from build123d import *

# Parameters (mm, degrees)
F0_W     = 56
F0_H     = 30
F0_R     = 5
F1_DEPTH = 15
F2_W     = 56
F2_H     = 15
F3_DEPTH = 18
F4_W     = 15
F4_H     = 5
F5_DEPTH = 25
F6_W     = 2
F6_H     = 15
F7_DEPTH = 20
F8_W     = 12
F8_H     = 15
F9_DEPTH = 20


with BuildPart() as f1:
    # F0 (on Top) → F1 (new body)
    with BuildSketch(Plane.XY):
        Rectangle(F0_W, F0_H)
        Circle(F0_R, mode=Mode.SUBTRACT)
    extrude(amount=F1_DEPTH)

    # F2 (on face) → F3 (cut)
    with BuildSketch(Plane.XZ.offset(15)):
        with Locations((0, 7.5)):
            Rectangle(F2_W, F2_H)
    extrude(amount=-F3_DEPTH, mode=Mode.SUBTRACT)

    # F4 (on face) → F5 (cut)
    with BuildSketch(Plane(origin=(0, 15, 0), x_dir=(-1, 0, 0), z_dir=(0, 1, 0))):
        with Locations((17.5, 7.5)):
            Rectangle(F4_W, F4_H)
    extrude(amount=-F5_DEPTH, mode=Mode.SUBTRACT)

    # F6 (on face) → F7 (cut)
    with BuildSketch(Plane(origin=(-28, 0, 0), x_dir=(0, -1, 0), z_dir=(-1, 0, 0))):
        with Locations((-4, 7.5)):
            Rectangle(F6_W, F6_H)
    extrude(amount=-F7_DEPTH, mode=Mode.SUBTRACT)

    # F8 (on face) → F9 (cut)
    with BuildSketch(Plane.YZ.offset(28)):
        with Locations((9, 7.5)):
            Rectangle(F8_W, F8_H)
    extrude(amount=-F9_DEPTH, mode=Mode.SUBTRACT)


solid = f1.part
Can you work these out from the model? Positions are in its coordinate system, mm. A direction names the side the tool comes from. Round coordinates to 2 decimals unless told otherwise and drop trailing zeros. Order: outer loops, then holes, each group sorted by start corner. A loop starts at its lowest first (then second) coordinate and runs counter-clockwise, first axis right, second up. Notation, with made-up numbers: M 35.25,7.25 L 40.25,7.25 A8 cw 40.25,14.25 Z; hole C 85.25,45.25 d5. An arc over 180 degrees is marked long. Use a Markdown table: item, result.
1) I'm going to push flat-ended pins straight in: P1, Ø2, axis at x = -22.5, z = 12.5, coming from the -Y side; P2, Ø1.6, axis at y = 4, z = 5, coming from the -X side; P3, Ø1, axis at x = -1.5, z = 8.5, coming from the -Y side. Where does each tip first touch, or does it pass through?
Geometry says:
| item | result |
|---|---|
| P1 | stops at y = 5 |
| P2 | stops at x = -8 |
| P3 | stops at y = 4.58 |
2) Imagine slicing it at A-A (x = -18). List the corners of the cut face in (y, z) for me.
Geometry says:
| item | result |
|---|---|
| outline | M 5,0 L 15,0 L 15,5 L 5,5 Z; M 5,10 L 15,10 L 15,15 L 5,15 Z |
3) Imagine slicing it at C-C (y = 7.25). List the corners of the cut face in (x, z) for me, then the cut area to 3 significant figures.
Geometry says:
| item | result |
|---|---|
| outline | M -28,0 L 8,0 L 8,15 L -28,15 Z; hole M -25,5 L -10,5 L -10,10 L -25,10 Z |
| area | 465 mm² |
4) Imagine slicing it at B-B (z = 7.25). List the corners of the cut face in (x, y) for me.
Geometry says:
| item | result |
|---|---|
| outline | M -28,5 L -25,5 L -25,15 L -28,15 Z; M -10,5 L -8,5 L -8,3 L -4,3 A5 cw 4,3 L 8,3 L 8,15 L -10,15 Z |
5) If we mould it in two halves opening along Z, with no side actions, what happens to faces 4 (the face through (-10, 9, 0)), 5 (the face through (-10, 9, 15)), 6 (the face through (8, 9, 8)), 7 (the face through (-10, 10, 7))? For each: +Z half, -Z half, draft (parallel to the pull), parting line (faces both ways), or undercut.
Geometry says:
| item | result |
|---|---|
| face 4 | -Z half |
| face 5 | +Z half |
| face 6 | draft |
| face 7 | undercut |
6) Imagine slicing it at D-D (z = 12). List the corners of the cut face in (x, y) for me.
Geometry says:
| item | result |
|---|---|
| outline | M -28,5 L -8,5 L -8,3 L -4,3 A5 cw 4,3 L 8,3 L 8,15 L -28,15 Z |
7) On a 3-axis mill with a long thin cutter (end or side, diameter ignored), from which of +Z, -Z, +X, -X, +Y, -Y can I reach the whole of each face in a straight line? I mean faces 1 (the face through (-18, 5, 4)), 2 (the face through (-17, 10, 5)), 3 (the face through (6, 3, 8)). Say none if no direction works.
Geometry says:
| item | result |
|---|---|
| face 1 | +Z, -Z, -X, -Y |
| face 2 | +Y, -Y |
| face 3 | +Z, -Z, +X, -X, -Y |
8) If I drill on line 1 along Z through (x, y) = (-21, 10.5); line 2 along X through (y, z) = (6.25, 9.75); line 3 along Y through (x, z) = (-18, 1), over which ranges is the centre line in solid material (lowest first)?
Geometry says:
| item | result |
|---|---|
| line 1 | z = 0 to 5, 10 to 15 |
| line 2 | x = -28 to -25, -10 to 8 |
| line 3 | y = 5 to 15 |
